Read the model definition and answer for the solid it produces. Units are mm, in the model's axes. A direction names the side the tool comes from. Give positions to 0.01 mm unless a question says otherwise; leave off trailing zeros. Order: outer loops, then holes, each group sorted by start corner. A loop starts at its lowest first (then second) coordinate and runs counter-clockwise, first axis right, second up. Notation, with made-up numbers: (-12.75, -7) - (14.25, -7) arc R14 cw to (14.25, 9) - close; hole circle Ø8 at (84, 10). An arc over 180 degrees is marked (long way). Return JSON: item names as keys, results as strings.
```python
from build123d import *

# Parameters (mm, degrees)
SKETCH1_W           = 44.45
SKETCH1_H           = 44.45
BOSS_EXTRUDE1_DEPTH = 3.175
BOSS_EXTRUDE2_DEPTH = 50.8
FILLET1_R           = 3.175
FILLET2_R           = 1.5875
FILLET3_R           = 3.175
SKETCH4_R           = 2.4892
CUT_EXTRUDE1_DEPTH  = 66.222877505
SKETCH5_W           = 15.875
SKETCH5_H           = 38.1
CUT_EXTRUDE2_DEPTH  = 64.515137759
FILLET4_R           = 7.9375
FILLET5_R           = 7.9375
CHAMFER1_SIZE       = 1.5875


with BuildPart() as part:
    # Sketch1 → Boss-Extrude1 (new, symmetric)
    with BuildSketch(Plane(origin=(0, 0, 0), x_dir=(1, 0, 0), z_dir=(0, 1, 0))):
        Rectangle(SKETCH1_W, SKETCH1_H)
    extrude(amount=BOSS_EXTRUDE1_DEPTH, both=True)

    # Sketch3 → Boss-Extrude2 (add)
    with BuildSketch(Plane.XZ.offset(3.175)):
        Polygon((12.0674, 14.518814274), (2.8134, 14.31134463), (2.8134, -14.31134463), (12.0674, -14.518814274), (12.0674, -17.693814274), (-12.0674, -17.693814274), (-12.0674, -14.518814274), (-2.8134, -14.31134463), (-2.8134, 14.31134463), (-12.0674, 14.518814274), (-12.0674, 17.693814274), (12.0674, 17.693814274), align=None)
    extrude(amount=BOSS_EXTRUDE2_DEPTH)

    # Fillet1
    fillet1_edges = [part.edges().sort_by_distance(p)[0] for p in [
        (22.225, 0, 22.225),
        (-22.225, 0, 22.225),
        (-22.225, 0, -22.225),
        (22.225, 0, -22.225),
    ]]
    fillet(fillet1_edges, radius=FILLET1_R)

    # Fillet2
    fillet2_edges = [part.edges().sort_by_distance(p)[0] for p in [
        (12.0674, -28.575, 17.693814274),
        (-12.0674, -28.575, 17.693814274),
        (-12.0674, -28.575, -17.693814274),
        (12.0674, -28.575, -17.693814274),
    ]]
    fillet(fillet2_edges, radius=FILLET2_R)

    # Fillet3
    fillet3_edges = [part.edges().sort_by_distance(p)[0] for p in [
        (7.4404, -3.175, -14.415079452),
        (2.8134, -3.175, 0),
        (7.4404, -3.175, 14.415079452),
        (-7.4404, -3.175, 14.415079452),
        (-2.8134, -3.175, 0),
        (-7.4404, -3.175, -14.415079452),
    ]]
    fillet(fillet3_edges, radius=FILLET3_R)

    # Sketch4 → Cut-Extrude1 (cut, through all)
    with BuildSketch(Plane(origin=(0, 3.175, 0), x_dir=(1, 0, 0), z_dir=(0, 1, 0))):
        with Locations(Location((17.4625, 17.4625, 0), (0, 0, 270))):
            Circle(SKETCH4_R)
        with Locations(Location((17.4625, -17.4625, 0), (0, 0, 270))):
            Circle(SKETCH4_R)
        with Locations(Location((-17.4625, -17.4625, 0), (0, 0, 270))):
            Circle(SKETCH4_R)
        with Locations(Location((-17.4625, 17.4625, 0), (0, 0, 270))):
            Circle(SKETCH4_R)
    extrude(amount=-CUT_EXTRUDE1_DEPTH, mode=Mode.SUBTRACT)

    # Sketch5 → Cut-Extrude2 (cut, through all)
    with BuildSketch(Plane(origin=(2.8134, 0, 0), x_dir=(0, 0, -1), z_dir=(1, 0, 0))):
        with Locations((0, -34.925)):
            Rectangle(SKETCH5_W, SKETCH5_H)
    extrude(amount=-CUT_EXTRUDE2_DEPTH, mode=Mode.SUBTRACT)

    # Fillet4
    fillet4_edges = [part.edges().sort_by_distance(p)[0] for p in [
        (0, -15.875, -7.9375),
        (0, -15.875, 7.9375),
    ]]
    fillet(fillet4_edges, radius=FILLET4_R - 0.0001)  # a hair under: the kernel refuses the full size

    # Fillet5
    fillet5_edges = [part.edges().sort_by_distance(p)[0] for p in [
        (0, -53.975, -7.9375),
        (0, -53.975, 7.9375),
    ]]
    fillet(fillet5_edges, radius=FILLET5_R)

    # Chamfer1
    chamfer1_edges = [part.edges().sort_by_distance(p)[0] for p in [
        (0, -3.175, -22.225),
        (22.225, -3.175, 0),
        (0, -3.175, 22.225),
        (-22.225, -3.175, 0),
        (21.29506403, -3.175, 21.29506403),
        (-21.29506403, -3.175, 21.29506403),
        (-21.29506403, -3.175, -21.29506403),
        (21.29506403, -3.175, -21.29506403),
    ]]
    chamfer(chamfer1_edges, length=CHAMFER1_SIZE)


solid = part.part
```
Q1. A cutting plane is placed at A-A (y = -36). Write down the section's boundary in (x, z) (1 decimal), and give its area (3 significant figures).
Values:
{"outline": "(-12.1, -16.1) arc R1.6 ccw to (-10.5, -17.7) - (10.5, -17.7) arc R1.6 ccw to (12.1, -16.1) - (12.1, -14.5) - (2.8, -14.3) - (2.8, -7.9) - (-2.8, -7.9) - (-2.8, -14.3) - (-12.1, -14.5) - close; (-12.1, 14.5) - (-2.8, 14.3) - (-2.8, 7.9) - (2.8, 7.9) - (2.8, 14.3) - (12.1, 14.5) - (12.1, 16.1) arc R1.6 ccw to (10.5, 17.7) - (-10.5, 17.7) arc R1.6 ccw to (-12.1, 16.1) - close", "area": "229 mm²"}
Q2. A cutting plane is placed at C-C (y = -8). Write down the section's boundary in (x, z) (1 decimal), and give its area (3 significant figures).
Values:
{"outline": "(-12.1, -16.1) arc R1.6 ccw to (-10.5, -17.7) - (10.5, -17.7) arc R1.6 ccw to (12.1, -16.1) - (12.1, -14.5) - (2.8, -14.3) - (2.8, 14.3) - (12.1, 14.5) - (12.1, 16.1) arc R1.6 ccw to (10.5, 17.7) - (-10.5, 17.7) arc R1.6 ccw to (-12.1, 16.1) - (-12.1, 14.5) - (-2.8, 14.3) - (-2.8, -14.3) - (-12.1, -14.5) - close", "area": "318 mm²"}
Q3. Given pin 1 (5 mm diameter, centred on x = 13.5, z = 10.5, fed in from -Y); pin 2 (1.7 mm diameter, centred on x = 0, y = -31.5, fed in from +Z); pin 3 (12 mm diameter, centred on y = -32, z = 7.5, fed in from +X), each flat-ended and moving along its own axis, determine where each tip first touches the part or whether it passes through.
Values:
{"pin 1": "stops at y = -3.41", "pin 2": "stops at z = 17.69", "pin 3": "stops at x = 2.81"}
Q4. For faces 5 (the cylindrical face through (-7.4, -4.08, -13.46)), 6 (the cylindrical face through (-0.056, -52.246, -10.929)), 7 (the flat face through (12.067, -28, -15)), 8 (the cylindrical face through (7.53, -4.08, -13.46)), determine the directions among +Z, -Z, +X, -X, +Y, -Y from which every point of the face is accessible in a straight line to the end or side of a thin tool.
Values:
{"face 5": "-X, -Y", "face 6": "+X, -X, -Y", "face 7": "+Z, -Z, +X, -Y", "face 8": "+X, -Y"}
Q5. Consider L1, parallel to X at y = -1, z = 15.5 (3 decimals); L2, parallel to Y at x = 8, z = -15.5 (3 decimals); L3, parallel to Y at x = -9, z = 0 (3 decimals). Determine where each line is inside the solid, lowest interval first.
Values:
{"L1": "x = -22.225 to -18.994, -15.931 to 15.931, 18.994 to 22.225", "L2": "y = -53.966 to 3.175", "L3": "y = -3.175 to 3.175"}
Q6. Determine the mould class of faces 1 (the flat face through (0, -53.975, 17)), 2 (the cylindrical face through (18.21, 0.04, -15.09)), 3 (the flat face through (-12.067, -28, -15)), 4 (the flat face through (22.225, 1, 0)) for opening direction X: released by +X, released by -X, zero draft, split by the parting line, or undercut.
Values:
{"face 1": "zero draft", "face 2": "undercut", "face 3": "released by -X", "face 4": "released by +X"}
Q7. A cutting plane is placed at D-D (x = 16). Write down the section's boundary in (y, z) (1 decimal).
Values:
{"outline": "(-3.2, -20.6) - (-1.6, -22.2) - (3.2, -22.2) - (3.2, -19.5) - (-3.2, -19.5) - close; (-3.2, -15.4) - (3.2, -15.4) - (3.2, 15.4) - (-3.2, 15.4) - close; (-3.2, 19.5) - (3.2, 19.5) - (3.2, 22.2) - (-1.6, 22.2) - (-3.2, 20.6) - close"}
